from build123d import *

# Parameters (mm, degrees)
F_6_0MM_DOWEL_HOLE1_D = 6
CIRPATTERN1_COUNT     = 60


with BuildPart() as part:
    # Sketch1 → Revolve1 (revolve)
    with BuildSketch(Plane.XY, mode=Mode.PRIVATE) as revolve1_sk:
        Polygon((0, 31.746365559), (-8.5, 31.746365559), (-8.5, -58.253634441), (-75, -58.253634441), (-75, -63.253634441), (-57, -63.253634441), (-57, -83.253634441), (-8.5, -83.253634441), (-8.5, -253.253634441), (0, -253.253634441), align=None)
    revolve(revolve1_sk.sketch.rotate(Axis((0, -253.253634441, 0), (0, 1, 0)), 270), axis=Axis((0, -253.253634441, 0), (0, 1, 0)))

    # Ø6.0mm Dowel Hole1 (through all)
    with Locations(Plane(origin=(0, -58.253634441, 0), x_dir=(1, 0, 0), z_dir=(0, 1, 0))):
        with Locations((0, 75)):
            f_6_0mm_dowel_hole1 = Hole(F_6_0MM_DOWEL_HOLE1_D / 2)

    # CirPattern1: Ø6.0mm Dowel Hole1 ×60 about axis
    cirpattern1_axis = Axis((0, 0, 0), (0, 1, 0))
    for i in range(1, CIRPATTERN1_COUNT):
        add(f_6_0mm_dowel_hole1.rotate(cirpattern1_axis, i * 360 / CIRPATTERN1_COUNT), mode=Mode.SUBTRACT)


solid = part.part
Verification items for the finished model (mm, model axes). A direction names the side the tool comes from. Give positions to 0.01 mm unless a question says otherwise; leave off trailing zeros. Write each loop counter-clockwise with the first axis right and the second up, starting at its lowest first coordinate (ties: lowest second). Pieces come first, ordered by that corner, then holes. Notation, with made-up numbers: M -35.5,29.5 L 2.5,29.5 A25 cw 2.5,49.5 Z; hole C 87.25,-34.75 d1. An arc over 180 degrees is marked long. Use CSV: the item, a comma, the result in double quotes.
1) Go/stop test with flat-tipped pins: pin 1 Ø1.5 at (x, z) = (-23.5, 47) entering from +Y; pin 2 Ø12 at (x, z) = (0, -30) entering from -Y; pin 3 Ø1.5 at (y, z) = (-62, 0.5) entering from -X. Record where each tip stops, or that it passes through.
Final values:
pin 1,"y = -58.25"
pin 2,"y = -83.25"
pin 3,"x = -72.27"
2) Access from +Z, -Z, +X, -X, +Y, -Y to the whole of each face (thin tool, end or side, straight path). Record for faces 1 (the face through (0, -253.254, 0)), 2 (the face through (55.645, -73.394, 12.356)), 3 (the face through (-8.428, -13.884, 1.107)).
Final values:
face 1,"+Z, -Z, +X, -X, -Y"
face 2,"-Y"
face 3,"+Y"
3) Cross-section at C-C (y = -124.5). Enter the section's corners in (x, z), plus the area to 3 significant figures.
Final values:
outline,"C 0,0 d17"
area,"227 mm²"
4) Cross-section at A-A (x = 0). Enter the section's corners in (y, z), plus the area to 3 significant figures.
Final values:
outline,"M -253.25,-8.5 L -83.25,-8.5 L -83.25,-57 L -63.25,-57 L -63.25,-72 L -58.25,-72 L -58.25,-8.5 L 31.75,-8.5 L 31.75,8.5 L -58.25,8.5 L -58.25,72 L -63.25,72 L -63.25,57 L -83.25,57 L -83.25,8.5 L -253.25,8.5 Z"
area,"7,420 mm²"
5) Material ranges on line 1 along Y through (x, z) = (23, -62.5); line 2 along Y through (x, z) = (20.5, 23.5); line 3 along Z through (x, y) = (-33, -73), recorded low to high.
Final values:
line 1,"-63.25 to -58.25"
line 2,"-83.25 to -58.25"
line 3,"-46.48 to 46.48"
6) Cross-section at B-B (z = 0). Enter the section's corners in (x, y), plus the area to 3 significant figures.
Final values:
outline,"M -72,-63.25 L -57,-63.25 L -57,-83.25 L -8.5,-83.25 L -8.5,-253.25 L 8.5,-253.25 L 8.5,-83.25 L 57,-83.25 L 57,-63.25 L 72,-63.25 L 72,-58.25 L 8.5,-58.25 L 8.5,31.75 L -8.5,31.75 L -8.5,-58.25 L -72,-58.25 Z"
area,"7,420 mm²"
